```python
from build123d import *

# Parameters (mm, degrees)
SKETCH1_W                      = 140
SKETCH1_H                      = 200
BODY_DEPTH                     = 4
CABLE_CANAL_DEPTH              = 1
MOUNTING_SCREW_HOLES_OUTLINE_R = 2.25
MOUNTING_SCREW_HOLES_DEPTH     = 4


# Read off the part's stored shape, not the designer's step: mounting_screw_holes
with BuildPart() as part:
    # Sketch1 → body (new body)
    with BuildSketch(Plane.XY):
        Rectangle(SKETCH1_W, SKETCH1_H)
    extrude(amount=BODY_DEPTH)

    # Sketch2 → cable_canal (cut)
    with BuildSketch(Plane.XY.offset(4)):
        Polygon((-40, 100), (-40, 0), (-70, 0), (-70, -20), (-40, -20), (-40, -100), (-20, -100), (-20, 100), align=None)
    extrude(amount=-CABLE_CANAL_DEPTH, mode=Mode.SUBTRACT)

    # mounting_screw_holes outline → mounting_screw_holes (cut)
    with BuildSketch(Plane.XY):
        with Locations((65, 95)):
            Circle(MOUNTING_SCREW_HOLES_OUTLINE_R)
        with Locations((-65, -95)):
            Circle(MOUNTING_SCREW_HOLES_OUTLINE_R)
        with Locations((65, -95)):
            Circle(MOUNTING_SCREW_HOLES_OUTLINE_R)
        with Locations((-65, 95)):
            Circle(MOUNTING_SCREW_HOLES_OUTLINE_R)
    extrude(amount=MOUNTING_SCREW_HOLES_DEPTH, mode=Mode.SUBTRACT)


solid = part.part
```
Design review of the part built by this model. Coordinates are the model's own, in mm. Give positions to 0.01 mm unless a question says otherwise; leave off trailing zeros. Order: outer loops, then holes, each group sorted by start corner. A loop starts at its lowest first (then second) coordinate and runs counter-clockwise, first axis right, second up. Notation, with made-up numbers: (-8, -38) - (18, -38) arc R26 ccw to (18, -16) - close; hole circle Ø8 at (-3.5, 15.25). An arc over 180 degrees is marked (long way). Use a Markdown table: item, result. Add a question column.
(1) Add section B-B on y = -95. Give the boundary of the cut face in (x, z).
(2) Mouldability with a two-part tool opening along Y and no side actions: class faces 1 (the face through (-70, -1, 2)), 2 (the face through (63.214, -96.369, 1.972)), 3 (the face through (-1, 100, 2)) as +Y half, -Y half, draft (parallel to the pull), parting line (faces both ways), or undercut.
(3) Add section C-C on y = -54. Give the boundary of the cut face in (x, z).
(4) Add section D-D on x = -65. Give the boundary of the cut face in (y, z), then the cut area to 3 significant figures.
(5) Wall thickness on probe 1 along Y at (x, z) = (-65, 2.6); probe 2 along X at (y, z) = (-62, 3.5); probe 3 along Y at (x, z) = (-49, 3.25): over which ranges is each line inside the solid? List them lowest first. Write a range as [from, to].
(6) Add section A-A on x = 65. Give the boundary of the cut face in (y, z).
(7) Clearance check with a flat-ended pin moving along its axis: P1, Ø0.8, axis at y = -14.5, z = 3.5, coming from the -X side. State where the tip first meets the part, or that it passes through.
Report:
| question | item | result |
|---|---|---|
| 1 | outline | (-70, 0) - (-67.25, 0) - (-67.25, 4) - (-70, 4) - close; (-62.75, 0) - (62.75, 0) - (62.75, 4) - (-20, 4) - (-20, 3) - (-40, 3) - (-40, 4) - (-62.75, 4) - close; (67.25, 0) - (70, 0) - (70, 4) - (67.25, 4) - close |
| 2 | face 1 | draft |
| 2 | face 2 | undercut |
| 2 | face 3 | +Y half |
| 3 | outline | (-70, 0) - (70, 0) - (70, 4) - (-20, 4) - (-20, 3) - (-40, 3) - (-40, 4) - (-70, 4) - close |
| 4 | outline | (-100, 0) - (-97.25, 0) - (-97.25, 4) - (-100, 4) - close; (-92.75, 0) - (92.75, 0) - (92.75, 4) - (0, 4) - (0, 3) - (-20, 3) - (-20, 4) - (-92.75, 4) - close; (97.25, 0) - (100, 0) - (100, 4) - (97.25, 4) - close |
| 4 | area | 744 mm² |
| 5 | probe 1 | y = [-100, -97.25], [-92.75, 92.75], [97.25, 100] |
| 5 | probe 2 | x = [-70, -40], [-20, 70] |
| 5 | probe 3 | y = [-100, -20], [0, 100] |
| 6 | outline | (-100, 0) - (-97.25, 0) - (-97.25, 4) - (-100, 4) - close; (-92.75, 0) - (92.75, 0) - (92.75, 4) - (-92.75, 4) - close; (97.25, 0) - (100, 0) - (100, 4) - (97.25, 4) - close |
| 7 | P1 | stops at x = -20 |
